```python
from build123d import *

# Parameters (mm, degrees)
CROQUIS1_R              = 1.5
CROQUIS1_R_2            = 4
SALIENTE_EXTRUIR1_DEPTH = 4
CROQUIS2_R              = 10.5
CORTAR_EXTRUIR1_DEPTH   = 1.5
CROQUIS3_R              = 0.75
CORTAR_EXTRUIR2_DEPTH   = 10


with BuildPart() as part:
    # Croquis1 → Saliente-Extruir1 (new body)
    with BuildSketch(Plane(origin=(0, 0, 0), x_dir=(0, 0, -1), z_dir=(1, 0, 0))):
        with BuildLine():
            Line((-70.1875, 12.498593671), (29.79, 13.998424911))
            ThreePointArc((29.79, 13.998424911), (44, 0), (29.79, -13.998424911))
            Line((29.79, -13.998424911), (-70.1875, -12.498593671))
            ThreePointArc((-70.1875, -12.498593671), (-82.5, 0), (-70.1875, 12.498593671))
        make_face()
        with Locations((30, 0)):
            Circle(CROQUIS1_R, mode=Mode.SUBTRACT)
        with Locations((-70, 0)):
            Circle(CROQUIS1_R_2, mode=Mode.SUBTRACT)
    extrude(amount=SALIENTE_EXTRUIR1_DEPTH)

    # Croquis2 → Cortar-Extruir1 (cut)
    with BuildSketch(Plane(origin=(4, 0, 0), x_dir=(0, 0, -1), z_dir=(1, 0, 0))):
        with Locations((-70, 0)):
            Circle(CROQUIS2_R)
    extrude(amount=-CORTAR_EXTRUIR1_DEPTH, mode=Mode.SUBTRACT)

    # Croquis3 → Cortar-Extruir2 (cut)
    with BuildSketch(Plane.ZY):
        with Locations((63.65189161, -5.658093307)):
            Circle(CROQUIS3_R)
        with Locations((76.34810839, 5.658093307)):
            Circle(CROQUIS3_R)
        with Locations((64.341906693, 6.34810839)):
            Circle(CROQUIS3_R)
        with Locations((75.658093307, -6.34810839)):
            Circle(CROQUIS3_R)
    extrude(amount=-CORTAR_EXTRUIR2_DEPTH, mode=Mode.SUBTRACT)


solid = part.part
```
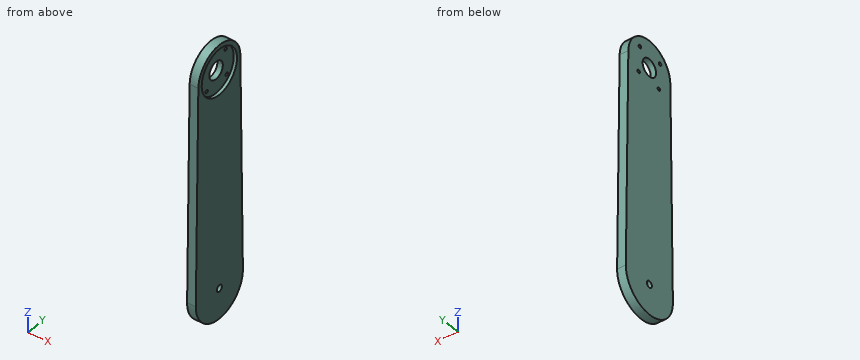
Read the model definition and answer for the solid it produces. Units are mm, in the model's axes. Give positions to 0.01 mm unless a question says otherwise; leave off trailing zeros. Order: outer loops, then holes, each group sorted by start corner. A loop starts at its lowest first (then second) coordinate and runs counter-clockwise, first axis right, second up.
(1) Find section B-B (x = 3.35). Give the vertices of the cut face in (y, z).
(2) Given pin 1 (2 mm diameter, centred on y = 5.66, z = 76.35, fed in from +X); pin 2 (2 mm diameter, centred on x = 3, z = -10, fed in from +Y); pin 3 (2 mm diameter, centred on x = 3.5, y = -6, fed in from +Z), each flat-ended and moving along its own axis, determine where each tip first touches the part or whether it passes through.
(3) Find section D-D (y = -8.75). Give the vertices of the cut face in (x, z).
(4) Find section C-C (z = 71.5). Give the vertices of the cut face in (x, y), plus the area to 3 significant figures.
(5) Straight lines are drawn through the part: L1, parallel to Y at x = 3.1, z = 70; L2, parallel to X at y = -0.5, z = 66; L3, parallel to Z at x = 2.9, y = 6.5. For each, find the intervals that lie inside material, in ascending order.
(6) Find section A-A (y = 0). Give the vertices of the cut face in (x, z).
Result sheet:
1. outline: (-14, -29.79) arc R14 ccw (long way) to (14, -29.79) - (12.5, 70.19) arc R12.5 ccw to (-12.5, 70.19) - close; hole circle Ø21 at (0, 70); hole circle Ø3 at (0, -30)
2. pin 1: stops at x = 2.5
2. pin 2: stops at y = 13.72
2. pin 3: stops at z = 81.46
3. outline: (0, -40.93) - (4, -40.93) - (4, 64.2) - (2.5, 64.2) - (2.5, 75.8) - (4, 75.8) - (4, 78.93) - (0, 78.93) - close
4. outline: (0, -12.41) - (4, -12.41) - (4, -10.39) - (2.5, -10.39) - (2.5, -3.71) - (0, -3.71) - close; (0, 3.71) - (2.5, 3.71) - (2.5, 10.39) - (4, 10.39) - (4, 12.41) - (0, 12.41) - close
4. area: 49.6 mm2
5. L1: y = -12.5 to -10.5, 10.5 to 12.5
5. L2: x = 0 to 2.5
5. L3: z = -42.4 to 61.75, 78.25 to 80.68
6. outline: (0, -44) - (4, -44) - (4, -31.5) - (0, -31.5) - close; (0, -28.5) - (4, -28.5) - (4, 59.5) - (2.5, 59.5) - (2.5, 66) - (0, 66) - close; (0, 74) - (2.5, 74) - (2.5, 80.5) - (4, 80.5) - (4, 82.5) - (0, 82.5) - close
